Autodesk Inventor part; units mm, degrees
ref_plane "YZ Plane" through (0, 0, 0) normal (1, 0, 0) x (0, 1, 0)
ref_plane "XZ Plane" through (0, 0, 0) normal (0, 1, 0) x (-1, 0, 0)
ref_plane "XY Plane" through (0, 0, 0) normal (0, 0, 1) x (1, 0, 0)
sketch "Skizze1" plane through (0, 0, 0) normal (1, 0, 0) x (0, 1, 0)
  line L0 (-270, 270) -> (270, 270)
  line L1 (270, 270) -> (270, -270)
  line L2 (270, -270) -> (-270, -270)
  line L3 (-270, -270) -> (-270, 270)
  line L4 (-378, 0) -> (378, 0)
  line L5 (0, -378) -> (0, 378)
  point P0 (0, 0)
  dimension "d0" = 540
  dimension "d1" = 540
extrude "Extrusion1" add sketch "Skizze1" along normal blind 18
sketch "Skizze2" plane through (18, 0, 0) normal (1, 0, 0) x (0, 0, -1)
  line L0 (-270, 270) -> (-270, -270)
  line L1 (-270, -270) -> (270, -270)
  line L2 (270, -270) -> (270, 270)
  line L3 (270, 270) -> (-270, 270)
  line L4 (-203, -203) -> (203, -203)
  line L5 (203, -203) -> (203, 203)
  line L6 (203, 203) -> (-203, 203)
  line L7 (-203, 203) -> (-203, -203)
  point P0 (0, 0)
  dimension "d4" = 67
  dimension "d5" = 67
  dimension "d6" = 67
  dimension "d7" = 67
extrude "Extrusion2" cut sketch "Skizze2" against normal blind 10 contours L7 L6 L5 L4
sketch "Skizze3" plane through (8, 0, 0) normal (1, 0, 0) x (0, 0, -1)
  line L0 (203, -203) -> (-203, -203)
  line L1 (203, 203) -> (203, -203)
  line L2 (-203, 203) -> (203, 203)
  line L3 (-203, -203) -> (-203, 203)
  line L4 (-193, -193) -> (193, -193)
  line L5 (193, -193) -> (193, 193)
  line L6 (193, 193) -> (-193, 193)
  line L7 (-193, 193) -> (-193, -193)
  point P0 (0, 0)
  dimension "d10" = 10
  dimension "d11" = 10
  dimension "d12" = 10
  dimension "d13" = 10
extrude "Extrusion3" cut sketch "Skizze3" against normal blind 8 contours L7 L6 L5 L4
sketch "Skizze6" plane through (0, 0, 0) normal (-1, 0, 0) x (0, 0, 1)
  line L0 (-193, -193) -> (-193, 193)
  line L1 (-193, 193) -> (193, 193)
  line L2 (193, 193) -> (193, -193)
  line L3 (193, -193) -> (-193, -193)
  line L4 (270, -270) -> (270, 270)
  line L5 (270, 270) -> (-270, 270)
  line L6 (-270, 270) -> (-270, -270)
  line L7 (-270, -270) -> (270, -270)
  line L8 (17.5, -201) -> (17.5, -210)
  line L9 (22, -201) -> (17.5, -201)
  line L10 (17.5, -210) -> (13, -210)
  line L11 (13, -197) -> (13, -210)
  line L12 (22, -197) -> (22, -201)
  line L13 (-200, -197) -> (200, -197)
  line L14 (11, -197) -> (11, -210)
  line L15 (2, -197) -> (2, -201)
  line L16 (6.5, -201) -> (2, -201)
  line L17 (6.5, -201) -> (6.5, -210)
  line L18 (11, -210) -> (6.5, -210)
  line L19 (-5, -197) -> (-5, -201)
  line L20 (-5, -201) -> (-9.5, -201)
  line L21 (-9.5, -201) -> (-9.5, -210)
  line L22 (-9.5, -210) -> (-14, -210)
  line L23 (-14, -197) -> (-14, -210)
  line L24 (-16, -197) -> (-16, -210)
  line L25 (-16, -210) -> (-20.5, -210)
  line L26 (-20.5, -201) -> (-20.5, -210)
  line L27 (-20.5, -201) -> (-25, -201)
  line L28 (-25, -197) -> (-25, -201)
  line L29 (-270, -270) -> (270, -270)
  line L30 (-25, -243) -> (-25, -193)
  line L31 (25, -243) -> (25, -193)
  line L32 (0, -378) -> (0, 378)
  line L33 (-378, 0) -> (378, 0)
  line L34 (25, -243) -> (-25, -243)
  line L35 (25, -193) -> (-25, -193)
  point P0 (0, 0)
  dimension "d34" = 50
  dimension "d37" = 50
chamfer "Fase1" distance 18 angle 45 1 edges at (0, -270, 0)
chamfer "Fase2" distance 18 angle 45 2 edges at (0, 270, 0) (0, 8.9997, 270)
extrude "Extrusion7" cut sketch "Skizze6" against normal blind 15 contours L0 L33 L32 L3 | L0 L1 L32 L33 | L3 L32 L13 L30 | L33 L2 L3 L32 | L32 L1 L2 L33 | L3 L31 L13 L32 | L13 L24 L25 L26 L27 L28 | L32 L34 L30 L27 L26 L25 L24 L13 L23 L22 L21 L20 L19 | L13 L15 L16 L17 L18 L14 L11 L10 L8 L9 L12 L31 L34 L32 | L19 L20 L21 L22 L23 L13 | L13 L14 L18 L17 L16 L15 | L12 L9 L8 L10 L11 L13
sketch "Skizze8" plane through (18, 0, 0) normal (1, 0, 0) x (0, 0, -1)
  point P0 (0, 0)
sketch "Skizze9" plane through (18, 0, 0) normal (1, 0, 0) x (0, 0, -1)
  line L0 (-270, -270) -> (270, -270)
  line L1 (270, 270) -> (270, -270)
  point P0 (0, 0)
  point P1 (237, -232)
  dimension "d40" = 38
  dimension "d41" = 33
hole "Bohrung2" at (18, -232, -237) direction (-1, 0, 0) diameter 20 depth 18 tip angle 118
properties part number "PV_Rahmen"
Part model, mm, in its own coordinate system. A direction names the side the tool comes from. Round coordinates to 2 decimals unless told otherwise and drop trailing zeros. Loops run counter-clockwise (first coordinate to the right, second up) from the corner with the lowest first, then second, coordinate; pieces in that order, holes last.
1. Slice it at C-C (x = 4.25). Give the cut face in (y, z).
Solutions:
outline: (-256.25, -270) - (256.25, -270) - (256.25, 256.25) - (-256.25, 256.25) - close; hole (-243, -25) - (-193, -25) - (-193, -193) - (193, -193) - (193, 193) - (-193, 193) - (-193, 25) - (-243, 25) - close; hole circle Ø20 at (-232, -237)
2. Drill centre lines: line 1 along Z through (x, y) = (13.5, -232); line 2 along Z through (x, y) = (10, -232); line 3 along Z through (x, y) = (9.75, 95). Where is each one in solid material? Low to high.
Solutions:
line 1: z = -270 to -247, -227 to -25, 25 to 265.5
line 2: z = -270 to -247, -227 to -25, 25 to 262
line 3: z = -270 to -203, 203 to 261.75
3. 3-axis set-ups, long thin cutter, end or side, ignore diameter. For faces 1 (the face through (8.874, -228.17, -246.237)), 2 (the face through (8, 196, 1)), 3 (the face through (7, -218, -25)): which of +Z, -Z, +X, -X, +Y, -Y reach the whole face in a straight line?
Solutions:
face 1: +X, -X
face 2: +X
face 3: -X
4. Two-plate mould, pull along Y, no slides. Class faces 4 (the face through (9, 261, 4)), 5 (the face through (7, -243, 0)), 6 (the face through (9, 4, -270)): pulls with the +Y half, pulls with the -Y half, needs draft (parallel to the pull), parting line crosses it, or undercut.
Solutions:
face 4: pulls with the +Y half
face 5: undercut
face 6: needs draft
5. Flat gauge pins, fed straight in: pin 1 (2.5 mm diameter, centred on x = 2.5, z = 95, fed in from +Y); pin 2 (5 mm diameter, centred on x = 15, z = -44, fed in from -Y); pin 3 (2.5 mm diameter, centred on x = 2.5, y = -8, fed in from +Z). Where does each tip first touch, or does it go through?
Solutions:
pin 1: stops at y = 255.75
pin 2: stops at y = -269.5
pin 3: stops at z = 255.75
